Verification items for the finished model (mm, model axes). Face numbers are marked on the shaded views. A direction names the side the tool comes from. Coordinates: 2 decimals unless noted, no trailing zeros. Order: outer loops, then holes, each group sorted by start corner. A loop starts at its lowest first (then second) coordinate and runs counter-clockwise, first axis right, second up. Notation, with made-up numbers: (64.25, 89) -> (116.25, 89) arc R12 ccw to (116.25, 97) -> close; hole circle Ø6 at (42.25, -16.75). An arc over 180 degrees is marked (long way). Write item = value, one per line. Start each with the question number.
1. Cross-section at B-B on x = 10.5. Record the cut outline in (y, z), plus the area to 3 significant figures.
2. Thickness scan on line 1 along Y through (x, z) = (5.75, -7.25); line 2 along X through (y, z) = (-3.85, -11); line 3 along Z through (x, y) = (19.75, -1.05). Record the ranges inside material, lowest first. Write a range as from..to.
3. Go/stop test with flat-tipped pins: P1, Ø1, axis at x = 12, z = -8.5, coming from the +Y side; P2, Ø1, axis at y = -4.5, z = -14, coming from the +X side; P3, Ø1.2, axis at x = 8, y = -2, coming from the -Z side. Record where each tip stops, or that it passes through.
4. Cross-section at C-C on z = -16.25. Record the cut outline in (x, y).
5. Cross-section at D-D on y = -1.7. Record the cut outline in (x, z).
6. Set-up check for the marked faces 1 and 2: record each of +Z, -Z, +X, -X, +Y, -Y from which the full face is reachable in a straight line by a thin tool's end or side.
Autodesk Inventor part; units mm, degrees
ref_plane "YZ Plane" through (0, 0, 0) normal (1, 0, 0) x (0, 1, 0)
ref_plane "XZ Plane" through (0, 0, 0) normal (0, 1, 0) x (-1, 0, 0)
ref_plane "XY Plane" through (0, 0, 0) normal (0, 0, 1) x (1, 0, 0)
sketch "Sketch1" plane through (0, 0, 0) normal (0, 0, 1) x (1, 0, 0)
  line L0 (0.5037, -0.606) -> (30.1037, -0.606)
  line L1 (30.1037, -0.606) -> (30.1037, -4.956)
  line L2 (30.1037, -4.956) -> (0.5037, -4.956)
  line L3 (0.5037, -4.956) -> (0.5037, -0.606)
  point P0 (0, 0)
  dimension "d1" = 4.35
  dimension "d2" = 29.6
extrude "Extrusion1" add sketch "Sketch1" along normal blind 2
sketch "Sketch2" plane through (0, 0, 0) normal (0, 0, -1) x (-1, 0, 0)
  line L0 (-30.1037, -4.956) -> (-0.5037, -4.956)
  line L1 (-0.5037, -4.956) -> (-0.5037, -2.956)
  line L2 (-0.5037, -2.956) -> (-30.1037, -2.956)
  line L3 (-30.1037, -2.956) -> (-30.1037, -4.956)
  line L4 (-0.5037, -4.956) -> (-30.1037, -4.956)
  line L5 (-30.1037, -4.956) -> (-30.1037, -0.606)
  dimension "d11" = 29.6
  dimension "d12" = 2
extrude "Extrusion2" add sketch "Sketch2" along normal blind 17.6
chamfer "Chamfer2" distance 1 angle 45 1 edges at (15.3037, -2.956, -17.6)
sketch "Sketch3" plane through (0.5037, -2.956, 0) normal (0, 1, 0) x (1, 0, 0)
  line L0 (29.6, 17.6) -> (0, 17.6)
  line L1 (29.6, 17.6) -> (26.6, 17.6)
  line L2 (26.6, 17.6) -> (26.6, 5)
  line L3 (26.6, 5) -> (29.6, 5)
  line L4 (29.6, 5) -> (29.6, 17.6)
  point P0 (-0.5037, 0)
  dimension "d16" = 3
  dimension "d17" = 12.6
extrude "Extrusion3" cut sketch "Sketch3" against normal through all
fillet "Fillet1" radius 3 1 edges at (27.1037, -3.956, -5)
properties part number "tray_3DPrint"
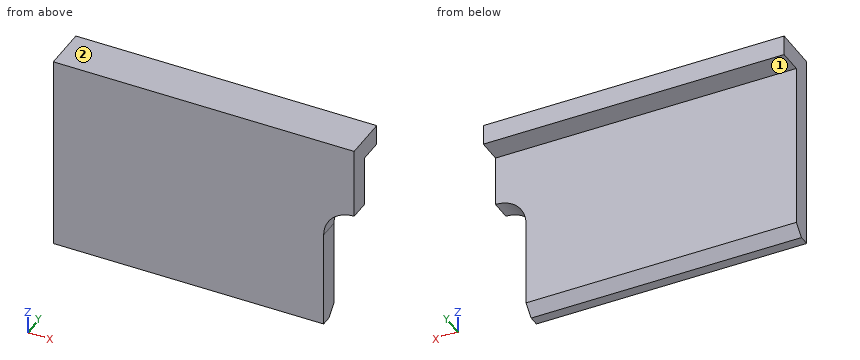
Worked out:
q1.outline = (-4.96, -17.6) -> (-3.96, -17.6) -> (-2.96, -16.6) -> (-2.96, 0) -> (-0.61, 0) -> (-0.61, 2) -> (-4.96, 2) -> close
q1.area = 43.4 mm²
q2.line_1 = -4.96..-2.96
q2.line_2 = 0.5..27.1
q2.line_3 = 0..2
q3.P1 = -2.96
q3.P2 = 27.1
q3.P3 = 0
q4.outline = (0.5, -4.96) -> (27.1, -4.96) -> (27.1, -2.96) -> (0.5, -2.96) -> close
q5.outline = (0.5, 0) -> (30.1, 0) -> (30.1, 2) -> (0.5, 2) -> close
q6.face_1 = -Z, +X, -X, +Y
q6.face_2 = +Z, +X, -X, +Y, -Y
